Can you work these out from the drawing? Everything is in mm from the part's minimum corner. Round coordinates to 2 decimals unless told otherwise and drop trailing zeros. Write each loop counter-clockwise with the first axis right and the second up, starting at its lowest first coordinate (ties: lowest second). Pieces come first, ordered by that corner, then holes. Notation, with made-up numbers: M 33.5,68 L 66.5,68 A29 cw 66.5,93 Z; hole C -16.75,-8.75 d7. An arc over 180 degrees is marked long. Use one line per item in the form item = value. Start each with the question number.
Q1. I want a section at A-A on y = 25.5. List the corners of the cut face in (x, z) for me, and give its area (3 significant figures).
Q2. We'd pull the mould along X, two halves only. Please class the marked faces 1, 2 and 3: +X half, -X half, draft (parallel to the pull), parting line (faces both ways), or undercut.
Q3. I want a section at C-C on x = 3. List the corners of the cut face in (y, z) for me, and give its area (3 significant figures).
Q4. I'm going to push a flat-ended pin straight in: pin 1 Ø2.5 at (x, y) = (3, 3.5) entering from +Z. Where does the tip first touch, or does it pass through?
Q5. I need wall thicknesses on line 1 along Y through (x, z) = (3, 1.5); line 2 along Y through (x, z) = (4.25, 2.4); line 3 along X through (y, z) = (24.5, 0.45). Which ranges of each line are inside material? Lowest first, please. Write a range as from..to.
Q6. I want a section at B-B on z = 1.9. List the corners of the cut face in (x, y) for me, and give its area (3 significant figures).
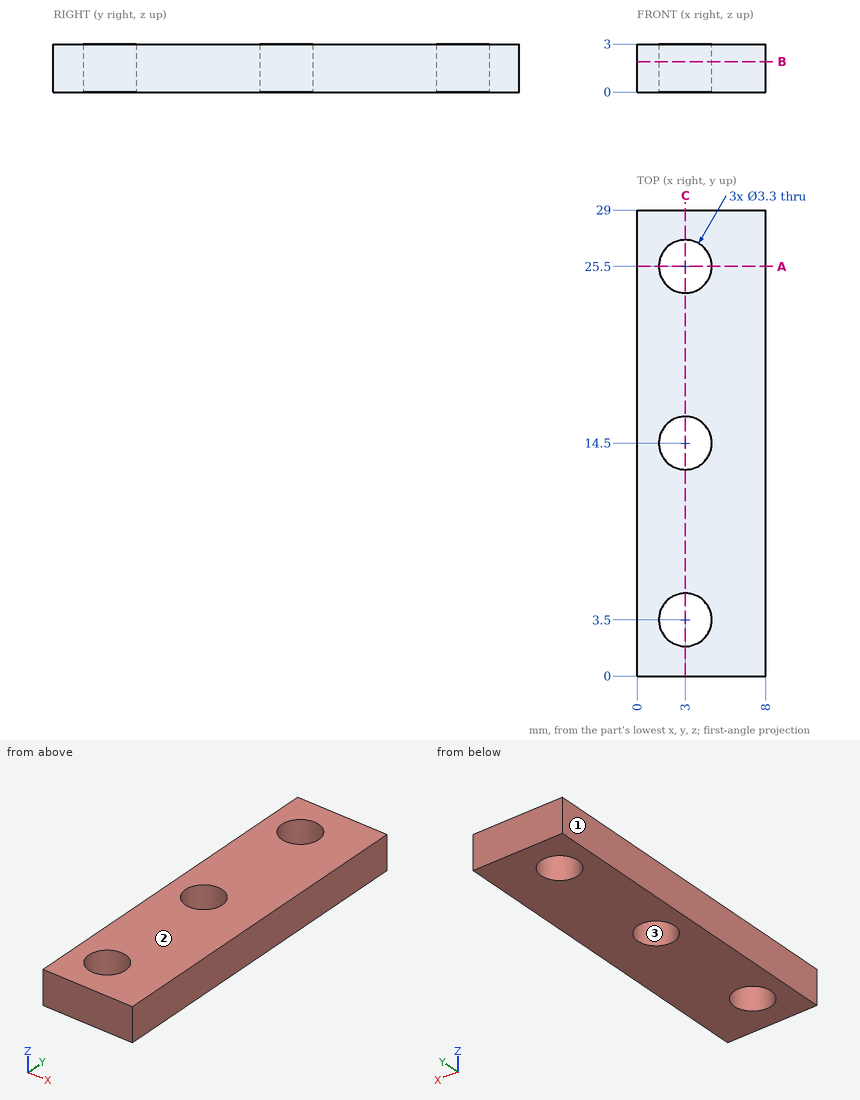
Reported:
q1.outline = M 0,0 L 1.35,0 L 1.35,3 L 0,3 Z; M 4.65,0 L 8,0 L 8,3 L 4.65,3 Z
q1.area = 14.1 mm^2
q2.face_1 = -X half
q2.face_2 = draft
q2.face_3 = undercut
q3.outline = M 0,0 L 1.85,0 L 1.85,3 L 0,3 Z; M 5.15,0 L 12.85,0 L 12.85,3 L 5.15,3 Z; M 16.15,0 L 23.85,0 L 23.85,3 L 16.15,3 Z; M 27.15,0 L 29,0 L 29,3 L 27.15,3 Z
q3.area = 57.3 mm^2
q4.pin_1 = through
q5.line_1 = 0..1.85, 5.15..12.85, 16.15..23.85, 27.15..29
q5.line_2 = 0..2.42, 4.58..13.42, 15.58..24.42, 26.58..29
q5.line_3 = 0..1.69, 4.31..8
q6.outline = M 0,0 L 8,0 L 8,29 L 0,29 Z; hole C 3,3.5 d3.3; hole C 3,14.5 d3.3; hole C 3,25.5 d3.3
q6.area = 206 mm^2
